from build123d import *

# Parameters (mm, degrees)
F1_DEPTH = 8.5
F3_DEPTH = 1.5
F4_R     = 4
F5_DEPTH = 1.5


with BuildPart() as f1:
    # F0 (on Top) → F1 (new body)
    with BuildSketch(Plane.XY):
        with BuildLine():
            ThreePointArc((24.8425577786, 1.8999753835), (14.7557370554, 8.519228761), (14.066705838, 20.5642984395))
            ThreePointArc((14.066705838, 20.5642984395), (0, 42), (-14.066705838, 20.5642984395))
            ThreePointArc((-14.066705838, 20.5642984395), (-14.7557370554, 8.519228761), (-24.8425577786, 1.8999753835))
            ThreePointArc((-24.8425577786, 1.8999753835), (-36.3730669589, -21), (-10.7758519407, -22.464273823))
            ThreePointArc((-10.7758519407, -22.464273823), (0, -17.038457522), (10.7758519407, -22.464273823))
            ThreePointArc((10.7758519407, -22.464273823), (36.3730669589, -21), (24.8425577786, 1.8999753835))
        make_face()
        with BuildLine():
            ThreePointArc((-12.23191812, 21.3602595126), (0, 40), (12.23191812, 21.3602595126))
            ThreePointArc((12.23191812, 21.3602595126), (13.0236862478, 7.519228761), (24.6144864293, -0.0869779274))
            ThreePointArc((24.6144864293, -0.0869779274), (34.6410161514, -20), (12.3825683094, -21.2732815852))
            ThreePointArc((12.3825683094, -21.2732815852), (0, -15.038457522), (-12.3825683094, -21.2732815852))
            ThreePointArc((-12.3825683094, -21.2732815852), (-34.6410161514, -20), (-24.6144864293, -0.0869779274))
            ThreePointArc((-24.6144864293, -0.0869779274), (-13.0236862478, 7.519228761), (-12.23191812, 21.3602595126))
        make_face(mode=Mode.SUBTRACT)
    extrude(amount=F1_DEPTH)

    # F2 (on face) → F3 (join)
    with BuildSketch(Plane.XY.offset(8.5)):
        with BuildLine():
            ThreePointArc((1.5, 39.9153563293), (0, 40), (-1.5, 39.9153563293))
            Line((-1.5, 39.9153563293), (-1.5, -15.1116190801))
            ThreePointArc((-1.5, -15.1116190801), (0, -15.038457522), (1.5, -15.1116190801))
            Line((1.5, -15.1116190801), (1.5, 39.9153563293))
        make_face()
    extrude(amount=-F3_DEPTH)

    # F4 (on face) → F5 (join, symmetric)
    with BuildSketch(Plane(origin=(0, 0, 7), x_dir=(1, 0, 0), z_dir=(0, 0, -1))):
        Circle(F4_R)
    extrude(amount=F5_DEPTH, both=True)


solid = f1.part
Can you work these out from the model? Positions are in its coordinate system, mm. A direction names the side the tool comes from. Coordinates: 2 decimals unless noted, no trailing zeros. Loops run counter-clockwise (first coordinate to the right, second up) from the corner with the lowest first, then second, coordinate; pieces in that order, holes last. Notation, with made-up numbers: (88, -17) - (111, -17) arc R18 ccw to (111, 8) - close; hole circle Ø10 at (53.25, -38.75). An arc over 180 degrees is marked (long way). Answer as a JSON object with one key per item and string values. Group by question number.
Item 1: If we section it at A-A (x = -6.5): List the corners of the cut face in (y, z) for me.
Item 2: If we section it at B-B (y = 16): List the corners of the cut face in (x, z) for me, plus the area to 3 significant figures.
Item 3: If we section it at C-C (z = 1.25): List the corners of the cut face in (x, y) for me, plus the area to 3 significant figures.
Item 4: On a 3-axis mill with a long thin cutter (end or side, diameter ignored), from which of +Z, -Z, +X, -X, +Y, -Y can I reach the whole of each face in a straight line? I mean faces 4 (the face through (-0.18, -17.04, 4.19)), 5 (the face through (0, 0, 5.5)), 6 (the face through (-13.125, 7.346, 4.19)). Say none if no direction works.
Item 5: If we mould it in two halves opening along X, with no side actions, what happens to faces 1 (the face through (14.844, 8.368, 4.19)), 2 (the face through (0, 4, 8.5)), 3 (the face through (3.695, 1.532, 6.979))? For each: released by +X, released by -X, zero draft, split by the parting line, or undercut.
Item 6: For pin 1 (2 mm diameter, centred on x = 5, z = 6.5, fed in from -Y); pin 2 (1 mm diameter, centred on x = -26.5, z = 5.5, fed in from +Y); pin 3 (3.5 mm diameter, centred on x = 0, y = 13.5, fed in from -Z), each with a flat end and sliding along its axis, tell me the tip position at first contact or that it passes through.
Item 7: If I drill on L1, parallel to Y at x = 0, z = 4; L2, parallel to X at y = -3, z = 6.5; L3, parallel to Y at x = 0, z = 6, over which ranges is the centre line in solid material (lowest first)? Write a range as from..to.
Item 8: If we section it at D-D (x = -30.5): List the corners of the cut face in (y, z) for me, plus the area to 3 significant figures.
Returned:
{
 "1": {"outline": "(-18.72, 0) - (-16.48, 0) - (-16.48, 8.5) - (-18.72, 8.5) - close; (38.31, 0) - (40.55, 0) - (40.55, 8.5) - (38.31, 8.5) - close"},
 "2": {"outline": "(-12.98, 0) - (-10.98, 0) - (-10.98, 8.5) - (-12.98, 8.5) - close; (-1.5, 7) - (1.5, 7) - (1.5, 8.5) - (-1.5, 8.5) - close; (10.98, 0) - (12.98, 0) - (12.98, 8.5) - (10.98, 8.5) - close", "area": "38.5 mm²"},
 "3": {"outline": "(-24.84, 1.9) arc R15.33 ccw (long way) to (-10.78, -22.46) arc R13.41 cw to (10.78, -22.46) arc R15.33 ccw (long way) to (24.84, 1.9) arc R13.41 cw to (14.07, 20.56) arc R15.33 ccw (long way) to (-14.07, 20.56) arc R13.41 cw to start; hole (-24.61, -0.09) arc R13.33 ccw (long way) to (-12.38, -21.27) arc R15.41 cw to (12.38, -21.27) arc R13.33 ccw (long way) to (24.61, -0.09) arc R15.41 cw to (12.23, 21.36) arc R13.33 ccw (long way) to (-12.23, 21.36) arc R15.41 cw to start", "area": "502 mm²"},
 "4": {"face 4": "+Z, -Z, -Y", "face 5": "-Z", "face 6": "+Z, -Z"},
 "5": {"face 1": "released by +X", "face 2": "zero draft", "face 3": "undercut"},
 "6": {"pin 1": "stops at y = -18.46", "pin 2": "stops at y = 1.72", "pin 3": "stops at z = 7"},
 "7": {"L1": "y = -17.04..-15.04, 40..42", "L2": "x = -34.42..-31.52, -2.65..2.65, 31.52..34.42", "L3": "y = -17.04..-15.04, -4..4, 40..42"},
 "8": {"outline": "(-26.76, 0) - (-24.42, 0) - (-24.42, 8.5) - (-26.76, 8.5) - close; (-2.25, 0) - (0.09, 0) - (0.09, 8.5) - (-2.25, 8.5) - close", "area": "39.8 mm²"}
}
